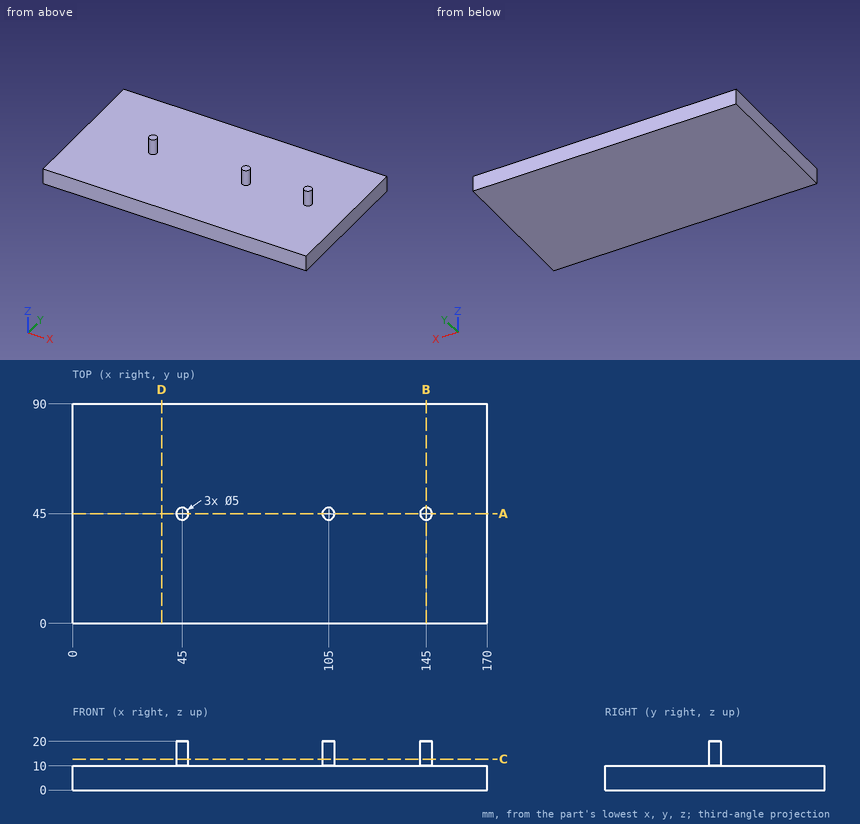
For this review, use the dimensioned drawing (mm, ordinates from the lowest corner) and the shaded views. Give positions to 0.01 mm unless a question says otherwise; leave off trailing zeros. Order: outer loops, then holes, each group sorted by start corner. A loop starts at its lowest first (then second) coordinate and runs counter-clockwise, first axis right, second up. Notation, with made-up numbers: (86.5, 79) - (119.5, 79) arc R16 ccw to (119.5, 101) - close; hole circle Ø11 at (88.25, 58). An arc over 180 degrees is marked (long way). Use CSV: the item, a comma, the result in double quotes. Start each with the question number.
Q1. Take a section at D-D (x = 36.5). State the section outline as (y, z) points.
Q2. For P1, Ø4, axis at x = 150.5, y = 50, coming from the +Z side; P2, Ø8, axis at y = 23, z = 17, coming from the +X side, all flat-tipped, find the tip position at first contact; note any pin that passes through.
Q3. Take a section at A-A (y = 45). State the section outline as (x, z) points.
Q4. Take a section at B-B (x = 145). State the section outline as (y, z) points.
Q5. Take a section at C-C (z = 12.75). State the section outline as (x, y) points, and give its area (3 significant figures).
Q6. For line 1 (Z direction, x = 82, y = 25); line 2 (Y direction, x = 145.5, z = 14); line 3 (Y direction, x = 146, z = 14), list the stretches that pass through material, from the lowest coordinate up.
Calculated:
1,outline,"(0, 0) - (90, 0) - (90, 10) - (0, 10) - close"
2,P1,"stops at z = 10"
2,P2,"passes through"
3,outline,"(0, 0) - (170, 0) - (170, 10) - (147.5, 10) - (147.5, 20) - (142.5, 20) - (142.5, 10) - (107.5, 10) - (107.5, 20) - (102.5, 20) - (102.5, 10) - (47.5, 10) - (47.5, 20) - (42.5, 20) - (42.5, 10) - (0, 10) - close"
4,outline,"(0, 0) - (90, 0) - (90, 10) - (47.5, 10) - (47.5, 20) - (42.5, 20) - (42.5, 10) - (0, 10) - close"
5,outline,"circle Ø5 at (45, 45); circle Ø5 at (105, 45); circle Ø5 at (145, 45)"
5,area,"58.9 mm²"
6,line 1,"z = 0 to 10"
6,line 2,"y = 42.55 to 47.45"
6,line 3,"y = 42.71 to 47.29"
